CAD build for the part. Positions are in the model's coordinates, mm. A direction names the side the tool comes from. Give positions to 0.01 mm unless a question says otherwise; leave off trailing zeros. Loops run counter-clockwise (first coordinate to the right, second up) from the corner with the lowest first, then second, coordinate; pieces in that order, holes last. Notation, with made-up numbers: (-1, 35) -> (5, 35) arc R15 cw to (5, 39) -> close; hole circle Ø6 at (40.5, 75). An arc over 180 degrees is marked (long way). Use one line per item in the form item = value.
```python
from build123d import *

# Parameters (mm, degrees)
SKETCH2_W          = 5.5
SKETCH2_H          = 0.8
CUT_EXTRUDE1_DEPTH = 0.8


with BuildPart() as part:
    # Sketch1 → Revolve1 (revolve)
    with BuildSketch(Plane.XY, mode=Mode.PRIVATE) as revolve1_sk:
        Polygon((0, 0), (0, 2.75), (2, 2.75), (2, 1.5), (7, 1.5), (7, 0), align=None)
    revolve(revolve1_sk.sketch.rotate(Axis((7, 0, 0), (-1, 0, 0)), 90), axis=Axis((7, 0, 0), (-1, 0, 0)))

    # Sketch2 → Cut-Extrude1 (cut)
    with BuildSketch(Plane.ZY):
        Rectangle(SKETCH2_W, SKETCH2_H)
    extrude(amount=-CUT_EXTRUDE1_DEPTH, mode=Mode.SUBTRACT)


solid = part.part
```
1. Drop a flat-ended pin along its axis: P1, Ø0.6, axis at x = 0.5, z = 0.5, coming from the +Y side. Give the stop position or say it passes through.
Result sheet:
P1 = 2.74
2. Cut at C-C, the plane x = 6.25. Write the cut outline in (y, z), then the cut area to 3 significant figures.
Result sheet:
outline = circle Ø3 at (0, 0)
area = 7.07 mm^2
3. Cut at D-D, the plane x = 0.5. Write the cut outline in (y, z), then the cut area to 3 significant figures.
Result sheet:
outline = (-0.4, -2.72) -> (-0.4, 2.72) arc R2.75 ccw to start; (0.4, -2.72) arc R2.75 ccw to (0.4, 2.72) -> close
area = 19.4 mm^2
4. Tool access for faces 1 (the flat face through (0, -1, 0)), 2 (the cylindrical face through (4.54, -0.45, -1.43)): list every direction of +Z, -Z, +X, -X, +Y, -Y with a clear straight run to the whole face (end or side of a thin tool).
Result sheet:
face_1 = +Z, -Z, -X, +Y, -Y
face_2 = +X
5. Drill centre lines: line 1 (X direction, y = 1.95, z = 1.45); line 2 (X direction, y = 0, z = 2.05); line 3 (Y direction, x = 1.5, z = 1.85). Where is each one in solid material? Low to high.
Result sheet:
line_1 = 0 to 2
line_2 = 0.8 to 2
line_3 = -2.03 to 2.03
6. Cut at B-B, the plane z = 0. Write the cut outline in (x, y), then the cut area to 3 significant figures.
Result sheet:
outline = (0, -2.75) -> (2, -2.75) -> (2, -1.5) -> (7, -1.5) -> (7, 1.5) -> (2, 1.5) -> (2, 2.75) -> (0, 2.75) -> (0, 0.4) -> (0.8, 0.4) -> (0.8, -0.4) -> (0, -0.4) -> close
area = 25.4 mm^2
7. Cut at A-A, the plane y = 0. Write the cut outline in (x, z).
Result sheet:
outline = (0.8, -2.75) -> (2, -2.75) -> (2, -1.5) -> (7, -1.5) -> (7, 1.5) -> (2, 1.5) -> (2, 2.75) -> (0.8, 2.75) -> close
8. Mould opens along Y. For faces 3 (the flat face through (2, 1.2, -1.2)), 4 (the cylindrical face through (1.01, 1.05, -2.54)), 5 (the flat face through (0.8, 0, 0)) say: pulls with the +Y half, pulls with the -Y half, needs draft (parallel to the pull), parting line crosses it, or undercut.
Result sheet:
face_3 = needs draft
face_4 = parting line crosses it
face_5 = undercut
